CAD build for the part. Positions are in the model's coordinates, mm. A direction names the side the tool comes from. Round coordinates to 2 decimals unless told otherwise and drop trailing zeros. Loops run counter-clockwise (first coordinate to the right, second up) from the corner with the lowest first, then second, coordinate; pieces in that order, holes last. Notation, with made-up numbers: (24.25, -11) -> (34.25, -11) arc R20 ccw to (34.25, 27) -> close; hole circle Ø7 at (82.25, 74). An arc over 180 degrees is marked (long way). Answer as CSV lines item,"result".
```python
from build123d import *

# Parameters (mm, degrees)
F2_DEPTH = 15
F3_R     = 1.5
F4_DEPTH = 23.001
F5_R     = 3
F6_DEPTH = 4.5
F9_DEPTH = 4.3


with BuildPart() as f2:
    # F1 (on Front) → F2 (new body)
    with BuildSketch(Plane.XZ):
        Polygon((-82, 0), (-39.5, 0), (-39.5, 14.5), (-28.5, 14.5), (-28.5, 16.5), (-26.5, 16.5), (-26.5, 18.5), (-20, 18.5), (-20, 16.5), (-18, 16.5), (-18, 14.5), (0, 14.5), (18, 14.5), (18, 16.5), (20, 16.5), (20, 18.5), (26.5, 18.5), (26.5, 16.5), (28.5, 16.5), (28.5, 14.5), (39.5, 14.5), (39.5, 0), (82, 0), (38, 23), (0, 23), (-38, 23), align=None)
    extrude(amount=F2_DEPTH)

    # F3 (on Top) → F4 (cut, through all)
    with BuildSketch(Plane.XY):
        with Locations((71, -7.5)):
            Circle(F3_R)
        with Locations((-71, -7.5)):
            Circle(F3_R)
    extrude(amount=F4_DEPTH, mode=Mode.SUBTRACT)

    # F5 (on offset) → F6 (cut)
    with BuildSketch(Plane.XY.offset(8.6)):
        with Locations((-70.968017, -7.505668)):
            Circle(F5_R)
        with Locations((71.05542, -7.498881)):
            Circle(F5_R)
    extrude(amount=-F6_DEPTH, mode=Mode.SUBTRACT)

    # F8 (on offset) → F9 (join)
    with BuildSketch(Plane.XY.offset(23)):
        Polygon((38, -15), (38, -13.471063), (7.746612, -7.5), (38, -1.528937), (38, 0), (30.253388, 0), (0, -5.971063), (-30.253388, 0), (-38, 0), (-38, -1.528937), (-7.746612, -7.5), (-38, -13.471063), (-38, -15), (-30.253388, -15), (0, -9.028937), (30.253388, -15), align=None)
    extrude(amount=-F9_DEPTH)


solid = f2.part
```
Q1. Slice it at A-A, the plane z = 8.75. Give the cut face in (x, y), and give its area (3 significant figures).
Results:
outline,"(-65.26, -15) -> (-39.5, -15) -> (-39.5, 0) -> (-65.26, 0) -> close; (39.5, -15) -> (65.26, -15) -> (65.26, 0) -> (39.5, 0) -> close"
area,"773 mm2"
Q2. Probe L1, parallel to Y at x = -71, z = 2.65; L2, parallel to X at y = -6.75, z = 3; L3, parallel to X at y = -7.5, z = 2.75. List the from-to ranges inside material, lowest first. Write a range as [from, to].
Results:
L1,"[-15, -9], [-6, 0]"
L2,"[-76.26, -72.3], [-69.7, -39.5], [39.5, 69.7], [72.3, 76.26]"
L3,"[-76.74, -72.5], [-69.5, -39.5], [39.5, 69.5], [72.5, 76.74]"
Q3. Drop flat-ended pins along their axis: pin 1 Ø1.6 at (y, z) = (-5.5, 16) entering from -X; pin 2 Ø2 at (x, y) = (19.5, -4) entering from -Z; pin 3 Ø2 at (x, y) = (48.5, -13) entering from +Z; pin 4 Ø2.5 at (x, y) = (-71, -7.5) entering from -Z. Give the stop position or say it passes through.
Results:
pin 1,"x = -52.92"
pin 2,"z = 16.5"
pin 3,"z = 18.03"
pin 4,"through"
Q4. Slice it at C-C, the plane y = -13.5. Give the cut face in (x, z), and give its area (3 significant figures).
Results:
outline,"(-82, 0) -> (-39.5, 0) -> (-39.5, 14.5) -> (-28.5, 14.5) -> (-28.5, 16.5) -> (-26.5, 16.5) -> (-26.5, 18.5) -> (-20, 18.5) -> (-20, 16.5) -> (-18, 16.5) -> (-18, 14.5) -> (18, 14.5) -> (18, 16.5) -> (20, 16.5) -> (20, 18.5) -> (26.5, 18.5) -> (26.5, 16.5) -> (28.5, 16.5) -> (28.5, 14.5) -> (39.5, 14.5) -> (39.5, 0) -> (82, 0) -> (38, 23) -> (-38, 23) -> close"
area,"1,550 mm2"
Q5. Tool access for faces 4 (the flat face through (-39.5, -7, 7)), 5 (the flat face through (-70, -6, 4.1)), 6 (the flat face through (-61, -7, 0)): list every direction of +Z, -Z, +X, -X, +Y, -Y with a clear straight run to the whole face (end or side of a thin tool).
Results:
face 4,"-Z, +Y, -Y"
face 5,"+Z"
face 6,"-Z, +X, -X, +Y, -Y"
Q6. Slice it at D-D, the plane x = -71. Give the cut face in (y, z).
Results:
outline,"(-15, 0) -> (-9, 0) -> (-9, 4.1) -> (-10.51, 4.1) -> (-10.51, 5.75) -> (-15, 5.75) -> close; (-6, 0) -> (0, 0) -> (0, 5.75) -> (-4.51, 5.75) -> (-4.51, 4.1) -> (-6, 4.1) -> close"
Q7. Two-plate mould, pull along X, no slides. Class faces 1 (the flat face through (-1, -15, 17)), 2 (the flat face through (39.5, -7, 7)), 3 (the flat face through (-59.69, -7.4, 11.66)): pulls with the +X half, pulls with the -X half, needs draft (parallel to the pull), parting line crosses it, or undercut.
Results:
face 1,"needs draft"
face 2,"undercut"
face 3,"pulls with the -X half"
Q8. Slice it at B-B, the plane x = 71. Give the cut face in (y, z), and give its area (3 significant figures).
Results:
outline,"(-15, 0) -> (-9, 0) -> (-9, 4.1) -> (-10.5, 4.1) -> (-10.5, 5.75) -> (-15, 5.75) -> close; (-6, 0) -> (0, 0) -> (0, 5.75) -> (-4.5, 5.75) -> (-4.5, 4.1) -> (-6, 4.1) -> close"
area,"64.1 mm2"
